Check sheet for the modelled part. Datum: model origin and axes. Units: mm. Face numbers are marked on the shaded views. A direction names the side the tool comes from. Coordinates: 2 decimals unless noted, no trailing zeros. Order: outer loops, then holes, each group sorted by start corner. A loop starts at its lowest first (then second) coordinate and runs counter-clockwise, first axis right, second up.
1. Thickness scan on line 1 (Y direction, x = 0, z = 11.25); line 2 (Z direction, x = -0.5, y = 6); line 3 (X direction, y = 11, z = 37.5). Record the ranges inside material, lowest first.
2. Gauge pin test, flat ends, axial feed: pin 1 Ø7.5 at (x, y) = (0, 0) entering from -Z; pin 2 Ø4 at (y, z) = (7, 12.5) entering from -X; pin 3 Ø4 at (y, z) = (8.5, 35) entering from -X. Record the tip position at first contact, or that the pin passes through.
3. Cross-section at A-A (y = 0). Enter the section's corners in (x, z).
4. Set-up check for the marked faces 1 and 2: record each of +Z, -Z, +X, -X, +Y, -Y from which the full face is reachable in a straight line by a thin tool's end or side.
5. Cross-section at C-C (z = 11). Enter the section's corners in (x, y), then the cut area to 3 significant figures.
6. Draft check along Y on the marked faces 3, 4 and 5. Enter one of: released by +Y, released by -Y, zero draft, split by the parting line, or undercut.
7. Cross-section at D-D (y = 5.5). Enter the section's corners in (x, z).
```python
from build123d import *

# Parameters (mm, degrees)
F0_R     = 12.7
F1_DEPTH = 50.8
F2_DEPTH = 50.8
F3_R     = 6.35
F4_DEPTH = 25.4
F5_R     = 3.96875
F6_DEPTH = 25.4


with BuildPart() as f1:
    # F0 (on Top) → F1 (new body)
    with BuildSketch(Plane.XY):
        Circle(F0_R)
    extrude(amount=F1_DEPTH)

    # F0 (on Top) → F2 (join)
    with BuildSketch(Plane.XY):
        Circle(F0_R)
    extrude(amount=F2_DEPTH)

    # F3 (on face) → F4 (cut)
    with BuildSketch(Plane.XY.offset(50.8)):
        Circle(F3_R)
    extrude(amount=-F4_DEPTH, mode=Mode.SUBTRACT)

    # F5 (on face) → F6 (cut)
    with BuildSketch(Plane(origin=(0, 0, 0), x_dir=(1, 0, 0), z_dir=(0, 0, -1))):
        Circle(F5_R)
    extrude(amount=-F6_DEPTH, mode=Mode.SUBTRACT)


solid = f1.part
```
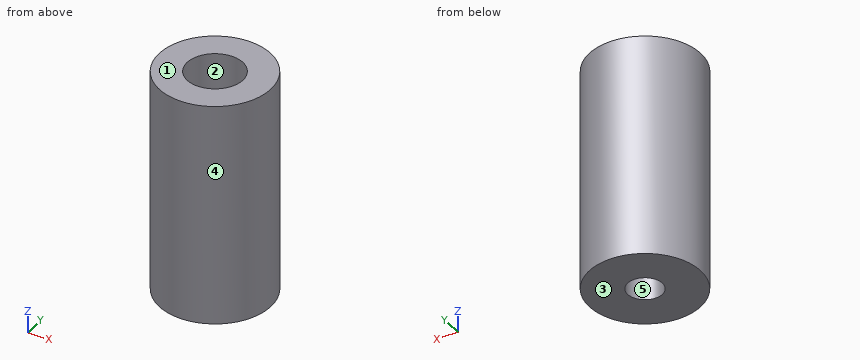
Data:
1. line 1: y = -12.7 to -3.97, 3.97 to 12.7
1. line 2: z = 0 to 25.4
1. line 3: x = -6.35 to 6.35
2. pin 1: passes through
2. pin 2: stops at x = -11.67
2. pin 3: stops at x = -10.91
3. outline: (-12.7, 0) - (-3.97, 0) - (-3.97, 25.4) - (-6.35, 25.4) - (-6.35, 50.8) - (-12.7, 50.8) - close; (3.97, 0) - (12.7, 0) - (12.7, 50.8) - (6.35, 50.8) - (6.35, 25.4) - (3.97, 25.4) - close
4. face 1: +Z, +X, -X, +Y, -Y
4. face 2: +Z
5. outline: circle Ø25.4 at (0, 0); hole circle Ø7.94 at (0, 0)
5. area: 457 mm2
6. face 3: zero draft
6. face 4: split by the parting line
6. face 5: undercut
7. outline: (-11.45, 0) - (11.45, 0) - (11.45, 50.8) - (3.17, 50.8) - (3.17, 25.4) - (-3.17, 25.4) - (-3.17, 50.8) - (-11.45, 50.8) - close
